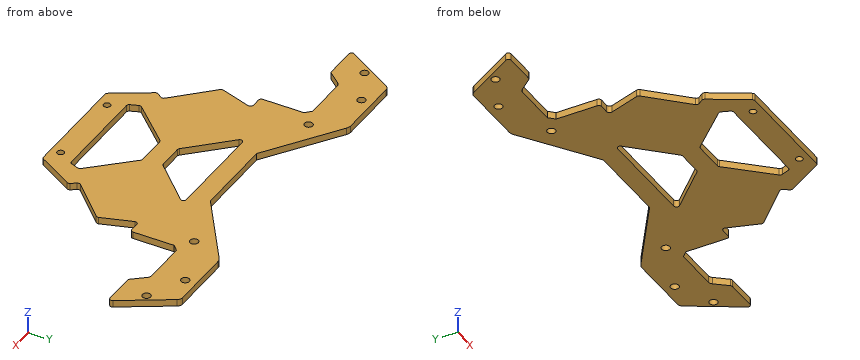
Autodesk Inventor part; units mm, degrees
ref_plane "YZ Plane" through (0, 0, 0) normal (1, 0, 0) x (0, 1, 0)
ref_plane "XZ Plane" through (0, 0, 0) normal (0, 1, 0) x (-1, 0, 0)
ref_plane "XY Plane" through (0, 0, 0) normal (0, 0, 1) x (1, 0, 0)
sketch "Sketch1" plane through (0, 0, 0) normal (0, 0, 1) x (1, 0, 0)
  line L0 (0, 76.5) -> (84, 76.5) construction
  line L1 (84, 76.5) -> (84, 0) construction
  line L2 (84, 0) -> (0, 0) construction
  line L3 (0, 0) -> (0, 76.5) construction
  line L4 (-37, 76.5) -> (0, 76.5) construction
  line L5 (0, 76.5) -> (0, 62) construction
  line L6 (0, 62) -> (-37, 62) construction
  line L7 (-37, 62) -> (-37, 76.5) construction
  line L8 (84, 76.5) -> (121, 76.5) construction
  line L9 (121, 76.5) -> (121, 62) construction
  line L10 (121, 62) -> (84, 62) construction
  line L11 (84, 62) -> (84, 76.5) construction
  line L12 (27, 58) -> (57, 58)
  line L13 (27, 58) -> (0.7665, 75.9748)
  line L14 (57, 58) -> (83.2335, 75.9748)
  line L15 (13.25, 14) -> (70.75, 14) construction
  line L16 (0, 76.5) -> (-25, 76.5) construction
  line L17 (-37, 76.5) -> (-37, 56.5) construction
  line L18 (-36.0913, 58.0145) -> (-25.5826, 75.529)
  line L19 (-35.2338, 56.5) -> (-23.9739, 56.5)
  line L20 (0, 62) -> (-19, 62) construction
  line L21 (-19.6002, 61.2665) -> (-23.1999, 56.8668)
  line L22 (0, 44) -> (84, 44) construction
  line L23 (1, 44) -> (4.371, 44)
  line L24 (83, 44) -> (79.629, 44)
  line L25 (1.5, 31) -> (82.5, 31) construction
  line L26 (5.3215, 42.6893) -> (1.6893, 31.579)
  line L27 (78.6785, 42.6893) -> (82.3107, 31.579)
  line L28 (15.3, 17) -> (68.7, 17) construction
  line L29 (82.0724, 30.5662) -> (69.278, 17.5864)
  line L30 (1.9276, 30.5662) -> (14.722, 17.5864)
  line L31 (69.1645, 16.3202) -> (70.3916, 14.5245)
  line L32 (14.8355, 16.3202) -> (13.6084, 14.5245)
  line L33 (21.5, 0) -> (62.5, 0) construction
  line L34 (21.2099, 0.4923) -> (13.5725, 13.4527)
  line L35 (62.7901, 0.4923) -> (70.4275, 13.4527)
  line L36 (84, 76.5) -> (109, 76.5) construction
  line L37 (121, 76.5) -> (121, 56.5) construction
  line L38 (120.0913, 58.0145) -> (109.5826, 75.529)
  line L39 (119.2338, 56.5) -> (107.9739, 56.5)
  line L40 (84, 62) -> (103, 62) construction
  line L41 (103.6002, 61.2665) -> (107.1999, 56.8668)
  line L42 (-23.8676, 76.5) -> (-0.9292, 76.5)
  line L43 (84.9292, 76.5) -> (107.8676, 76.5)
  line L44 (-18.0522, 62) -> (-2, 62)
  line L45 (102.0522, 62) -> (86, 62)
  line L46 (0, 60) -> (0, 45)
  line L47 (84, 60) -> (84, 45)
  line L48 (22.0714, 0) -> (61.9286, 0)
  line L49 (23.861, 51) -> (60.139, 51)
  line L50 (37.4235, 35) -> (46.5765, 35)
  line L51 (47.2947, 35.3042) -> (60.8572, 49.3042)
  line L52 (36.7053, 35.3042) -> (23.1428, 49.3042)
  line L53 (36.4346, 28) -> (47.5654, 28)
  line L54 (22, 13) -> (62, 13) construction
  line L55 (24.193, 9) -> (59.807, 9)
  line L56 (60.7433, 9.6489) -> (61.7824, 12.4197)
  line L57 (61.5771, 13.4531) -> (48.2965, 27.6823)
  line L58 (35.7035, 27.6823) -> (22.4229, 13.4531)
  line L59 (22.2176, 12.4197) -> (23.2567, 9.6489)
  line L60 (-28.5, 66) -> (112.5, 66) construction
  line L61 (-15, 72.5) -> (99, 72.5) construction
  line L62 (27, 3.5) -> (57, 3.5) construction
  arc A0 (0.7665, 75.9748) -> (-0.9292, 76.5) centre (-0.9292, 73.5) ccw
  arc A1 (84.9292, 76.5) -> (83.2335, 75.9748) centre (84.9292, 73.5) ccw
  arc A2 (-23.8676, 76.5) -> (-25.5826, 75.529) centre (-23.8676, 74.5) ccw
  arc A3 (109.5826, 75.529) -> (107.8676, 76.5) centre (107.8676, 74.5) ccw
  arc A4 (119.2338, 56.5) -> (120.0913, 58.0145) centre (119.2338, 57.5) ccw
  arc A5 (-36.0913, 58.0145) -> (-35.2338, 56.5) centre (-35.2338, 57.5) ccw
  arc A6 (-23.9739, 56.5) -> (-23.1999, 56.8668) centre (-23.9739, 57.5) ccw
  arc A7 (107.1999, 56.8668) -> (107.9739, 56.5) centre (107.9739, 57.5) ccw
  arc A8 (103.6002, 61.2665) -> (102.0522, 62) centre (102.0522, 60) ccw
  arc A9 (-18.0522, 62) -> (-19.6002, 61.2665) centre (-18.0522, 60) ccw
  line L63 (-2, 62) -> (0, 60)
  line L64 (84, 60) -> (86, 62)
  arc A10 (0, 45) -> (1, 44) centre (1, 45) ccw
  arc A11 (83, 44) -> (84, 45) centre (83, 45) ccw
  arc A12 (79.629, 44) -> (78.6785, 42.6893) centre (79.629, 43) ccw
  arc A13 (5.3215, 42.6893) -> (4.371, 44) centre (4.371, 43) ccw
  arc A14 (1.6893, 31.579) -> (1.9276, 30.5662) centre (2.6398, 31.2682) ccw
  arc A15 (82.0724, 30.5662) -> (82.3107, 31.579) centre (81.3602, 31.2682) ccw
  arc A16 (69.278, 17.5864) -> (69.1645, 16.3202) centre (69.9902, 16.8844) ccw
  arc A17 (70.4275, 13.4527) -> (70.3916, 14.5245) centre (69.5659, 13.9603) ccw
  arc A18 (61.9286, 0) -> (62.7901, 0.4923) centre (61.9286, 1) ccw
  arc A19 (21.2099, 0.4923) -> (22.0714, 0) centre (22.0714, 1) ccw
  arc A20 (13.6084, 14.5245) -> (13.5725, 13.4527) centre (14.4341, 13.9603) ccw
  arc A21 (14.8355, 16.3202) -> (14.722, 17.5864) centre (14.0098, 16.8844) ccw
  arc A22 (23.2567, 9.6489) -> (24.193, 9) centre (24.193, 10) ccw
  arc A23 (22.4229, 13.4531) -> (22.2176, 12.4197) centre (23.154, 12.7708) ccw
  arc A24 (36.4346, 28) -> (35.7035, 27.6823) centre (36.4346, 27) ccw
  arc A25 (48.2965, 27.6823) -> (47.5654, 28) centre (47.5654, 27) ccw
  arc A26 (61.7824, 12.4197) -> (61.5771, 13.4531) centre (60.846, 12.7708) ccw
  arc A27 (59.807, 9) -> (60.7433, 9.6489) centre (59.807, 10) ccw
  arc A28 (23.861, 51) -> (23.1428, 49.3042) centre (23.861, 50) ccw
  arc A29 (60.8572, 49.3042) -> (60.139, 51) centre (60.139, 50) ccw
  arc A30 (46.5765, 35) -> (47.2947, 35.3042) centre (46.5765, 36) ccw
  arc A31 (36.7053, 35.3042) -> (37.4235, 35) centre (37.4235, 36) ccw
  circle A32 centre (-15, 72.5) radius 1.5
  circle A33 centre (-28.5, 66) radius 1.5
  circle A34 centre (112.5, 66) radius 1.5
  circle A35 centre (99, 72.5) radius 1.5
  circle A36 centre (57, 3.5) radius 1.25
  circle A37 centre (27, 3.5) radius 1.25
  line L65 (5, 64.5) -> (79, 64.5) construction
  circle A38 centre (5, 64.5) radius 1.5
  circle A39 centre (79, 64.5) radius 1.5
  point P0 (-23.5, 56.5)
  point P1 (5.75, 44)
  point P2 (78.25, 44)
  point P3 (107.5, 56.5)
  point P4 (21.5, 51)
  point P5 (62.5, 51)
  point P6 (37, 35)
  point P7 (47, 35)
  point P8 (36, 28)
  point P9 (48, 28)
  point P10 (23.5, 9)
  point P11 (60.5, 9)
  dimension "d0" = 84
  dimension "d1" = 76.5
  dimension "d2" = 37
  dimension "d3" = 14.5
  dimension "d4" = 14.5
  dimension "d5" = 37
  dimension "d7" = 30
  dimension "d8" = 27
  dimension "d9" = 58
  dimension "d10" = 57.5
  dimension "d11" = 13.25
  dimension "d12" = 14
  dimension "d13" = 25
  dimension "d14" = 20
  dimension "d15" = 13.5
  dimension "d16" = 19
  dimension "d17" = 18
  dimension "d18" = 5.75
  dimension "d19" = 5.75
  dimension "d20" = 81
  dimension "d21" = 13
  dimension "d22" = 1.5
  dimension "d23" = 53.4
  dimension "d24" = 14
  dimension "d25" = 15.3
  dimension "d26" = 41
  dimension "d27" = 21.5
  dimension "d28" = 25
  dimension "d29" = 20
  dimension "d30" = 13.5
  dimension "d31" = 19
  dimension "d32" = 41
  dimension "d33" = 21.5
  dimension "d34" = 7
  dimension "d35" = 10
  dimension "d36" = 23
  dimension "d37" = 37
  dimension "d38" = 12
  dimension "d39" = 28
  dimension "d40" = 36
  dimension "d41" = 40
  dimension "d42" = 13
  dimension "d43" = 22
  dimension "d44" = 37
  dimension "d45" = 9
  dimension "d46" = 23.5
  dimension "d47" = 141
  dimension "d48" = 10.5
  dimension "d49" = 8.5
  dimension "d50" = 114
  dimension "d51" = 4
  dimension "d52" = 22
  dimension "d53" = 30
  dimension "d54" = 3.5
  dimension "d55" = 27
  dimension "d56" = 3
  dimension "d57" = 3
  dimension "d58" = 2
  dimension "d59" = 2
  dimension "d60" = 1
  dimension "d61" = 1
  dimension "d62" = 1
  dimension "d63" = 1
  dimension "d64" = 2
extrude "Extrusion3" add sketch "Sketch1" along normal blind 2.5
properties part number "RCT-H001_Al_side_plate"
Geometry check sheet. Reference: the model listing, model coordinates, mm. Round coordinates to 2 decimals unless told otherwise and drop trailing zeros. Order: outer loops, then holes, each group sorted by start corner. A loop starts at its lowest first (then second) coordinate and runs counter-clockwise, first axis right, second up. Notation, with made-up numbers: (65.5, 56.5) - (113.5, 56.5) arc R22 ccw to (113.5, 68.5) - close; hole circle Ø8 at (-40, 28). An arc over 180 degrees is marked (long way). Use a Markdown table: item, result. Add a question column.
(1) Sectioned sample at A-A, the plane x = 99. Enter the section's corners in (y, z).
(2) Sectioned sample at D-D, the plane x = 10.5. Enter the section's corners in (y, z).
(3) Sectioned sample at C-C, the plane z = 0.7. Count the separate pieces of the cut face and the enclosed holes in it, and give its area (3 significant figures).
(4) Sectioned sample at B-B, the plane x = 40.5. Enter the section's corners in (y, z), and give its area (3 significant figures).
(5) Material ranges on line 1 along Y through (x, z) = (32.5, 2.3); line 2 along X through (y, z) = (61.5, 1.35); line 3 along X through (y, z) = (11, 1.7), recorded low to high. Write a range as [from, to].
(6) Depth check by flat-ended pin: pin 1 (1.2 mm diameter, centred on x = 41.5, z = 0.5, fed in from +Y); pin 2 (1.2 mm diameter, centred on x = 81, z = 1.5, fed in from -Y); pin 3 (1 mm diameter, centred on y = 18.5, z = 1, fed in from -X). Enter the tip coordinate at first touch or a pass-through.
Answers below:
| question | item | result |
|---|---|---|
| 1 | outline | (62, 0) - (71, 0) - (71, 2.5) - (62, 2.5) - close; (74, 0) - (76.5, 0) - (76.5, 2.5) - (74, 2.5) - close |
| 2 | outline | (21.87, 0) - (69.31, 0) - (69.31, 2.5) - (21.87, 2.5) - close |
| 3 | separate pieces | 1 |
| 3 | enclosed holes | 10 |
| 3 | area | 4,480 mm² |
| 4 | outline | (0, 0) - (9, 0) - (9, 2.5) - (0, 2.5) - close; (28, 0) - (35, 0) - (35, 2.5) - (28, 2.5) - close; (51, 0) - (58, 0) - (58, 2.5) - (51, 2.5) - close |
| 4 | area | 57.5 mm² |
| 5 | line 1 | [0, 9], [24.25, 39.65], [51, 58] |
| 5 | line 2 | [-34, -19.38], [-1.5, 21.89], [62.11, 85.5], [103.38, 118] |
| 5 | line 3 | [15.02, 22.75], [61.25, 68.98] |
| 6 | pin 1 | y = 58 |
| 6 | pin 2 | y = 28.87 |
| 6 | pin 3 | x = 13.33 |
